Geometry check sheet. Reference: the model listing, model coordinates, mm. A direction names the side the tool comes from. Round coordinates to 2 decimals unless told otherwise and drop trailing zeros. Order: outer loops, then holes, each group sorted by start corner. A loop starts at its lowest first (then second) coordinate and runs counter-clockwise, first axis right, second up. Notation, with made-up numbers: (65, -31) -> (118, -31) arc R28 cw to (118, -3) -> close; hole circle Ø7 at (68, 29.5). An arc over 180 degrees is marked (long way). Answer as a JSON object with one key per item and string values. Group by question number.
from build123d import *

# Parameters (mm, degrees)
SHELL1_T  = -5
SKETCH3_W = 60
SKETCH3_H = 12


with BuildPart() as part:
    # Sketch2 → Revolve1 (revolve)
    with BuildSketch(Plane(origin=(0, 0, 0), x_dir=(1, 0, 0), z_dir=(0, 1, 0))):
        with BuildLine():
            Line((0, 25), (0, 0))
            Line((0, 0), (25, 0))
            ThreePointArc((25, 0), (17.67766953, 17.67766953), (0, 25))
        make_face()
    revolve(axis=Axis((0, 0, 0), (1, 0, 0)))

    # Shell1
    shell1_openings = [part.faces().sort_by_distance(p)[0] for p in [
        (0, 0, 25),
    ]]
    offset(amount=SHELL1_T, openings=shell1_openings, kind=Kind.INTERSECTION)

    # Sketch3 → Revolve3 (revolve)
    with BuildSketch(Plane.XY):
        with Locations((50, 6)):
            Rectangle(SKETCH3_W, SKETCH3_H)
    revolve(axis=Axis((20, 0, 0), (1, 0, 0)))


solid = part.part
Item 1: Sectioned sample at A-A, the plane z = 8.5. Enter the section's corners in (x, y).
Item 2: Set-up check for faces 1 (the flat face through (80, 0, 0)), 2 (the cylindrical face through (51.37, -11.99, 0.53)): record each of +Z, -Z, +X, -X, +Y, -Y from which the full face is reachable in a straight line by a thin tool's end or side.
Item 3: Depth check by flat-ended pin: pin 1 Ø5 at (x, y) = (66, -4) entering from +Z; pin 2 Ø3 at (y, z) = (7.5, 17) entering from +X; pin 3 Ø5 at (x, z) = (63.5, -5) entering from +Y. Enter the tip coordinate at first touch or a pass-through.
Item 4: Sectioned sample at B-B, the plane y = 0. Enter the section's corners in (x, z), then the cut area to 3 significant figures.
Item 5: Thickness scan on L1, parallel to Y at x = 73, z = 6.5; L2, parallel to Z at x = 4.5, y = -21.5; L3, parallel to X at y = 2, z = 17.5. Record the ranges inside material, lowest first.
Item 6: Sectioned sample at C-C, the plane x = 14.5. Enter the section's corners in (y, z).
Item 7: Sectioned sample at D-D, the plane x = 56.5. Enter the section's corners in (y, z), then the cut area to 3 significant figures.
Result:
{
 "1": {"outline": "(0, -23.51) arc R23.51 ccw to (21.93, -8.47) -> (80, -8.47) -> (80, 8.47) -> (21.93, 8.47) arc R23.51 ccw to (0, 23.51) -> (0, 18.1) arc R18.1 cw to (0, -18.1) -> close"},
 "2": {"face 1": "+Z, -Z, +X, +Y, -Y", "face 2": "+X"},
 "3": {"pin 1": "stops at z = 11.91", "pin 2": "stops at x = 18.25", "pin 3": "stops at y = 11.74"},
 "4": {"outline": "(0, -25) arc R25 ccw to (21.93, -12) -> (80, -12) -> (80, 12) -> (21.93, 12) arc R25 ccw to (0, 25) -> (0, 20) arc R20 cw to (0, -20) -> close", "area": "1,700 mm2"},
 "5": {"L1": "y = -10.09 to 10.09", "L2": "z = -11.94 to 11.94", "L3": "x = 9.47 to 17.74"},
 "6": {"outline": "circle Ø40.73 at (0, 0); hole circle Ø27.55 at (0, 0)"},
 "7": {"outline": "circle Ø24 at (0, 0)", "area": "452 mm2"}
}
